The model under review builds one solid part; all positions refer to its coordinate system, in mm. Face numbers are marked on the shaded views. A direction names the side the tool comes from. Coordinates: 2 decimals unless noted, no trailing zeros. Order: outer loops, then holes, each group sorted by start corner. A loop starts at its lowest first (then second) coordinate and runs counter-clockwise, first axis right, second up.
```python
from build123d import *

# Parameters (mm, degrees)
SKETCH_1_R          = 6
EXTRUDE_1_DEPTH     = 20
CUT_EXTRUDE_1_DEPTH = 8
CUT_EXTRUDE_START   = -6
SKETCH_3_R          = 6
SKETCH_3_R_2        = 4.1
CUT_EXTRUDE_2_DEPTH = 6
FILLET_1_R          = 1


with BuildPart() as part:
    # Эскиз1 → Вытянуть1 (new body)
    with BuildSketch(Plane(origin=(0, 0, 0), x_dir=(0, 0, -1), z_dir=(1, 0, 0))):
        Circle(SKETCH_1_R)
    extrude(amount=EXTRUDE_1_DEPTH)

    # Эскиз2 → Вырез-Вытянуть1 (cut)
    with BuildSketch(Plane.ZY):
        Polygon((-3, -1.732050808), (0, -3.464101615), (0, 3.464101615), (-3, 1.732050808), align=None)
        Polygon((0, -3.464101615), (0, 3.464101615), (3, 1.732050808), (3, -1.732050808), align=None)
    extrude(amount=-CUT_EXTRUDE_1_DEPTH, mode=Mode.SUBTRACT)

    # Эскиз3 → Вырез-Вытянуть2 (cut)
    with BuildSketch(Plane(origin=(20, 0, 0), x_dir=(0, 0, -1), z_dir=(1, 0, 0)).offset(CUT_EXTRUDE_START)):
        Circle(SKETCH_3_R)
        Circle(SKETCH_3_R_2, mode=Mode.SUBTRACT)
    extrude(amount=CUT_EXTRUDE_2_DEPTH, mode=Mode.SUBTRACT)

    # Эскиз4 → Вырез-Повернуть1 (revolve, cut)
    with BuildSketch(Plane.XY, mode=Mode.PRIVATE) as cut_revolve_1_sk:
        Polygon((14, 6), (14, 4.1), (12.1, 6), align=None)
    revolve(cut_revolve_1_sk.sketch.rotate(Axis((0, 0, 0), (1, 0, 0)), 90), axis=Axis((0, 0, 0), (1, 0, 0)), mode=Mode.SUBTRACT)

    # Эскиз5 → Вырез-Повернуть2 (revolve, cut)
    with BuildSketch(Plane.XY, mode=Mode.PRIVATE) as cut_revolve_2_sk:
        Polygon((0, 6), (0, 4.9), (1.1, 6), align=None)
    revolve(cut_revolve_2_sk.sketch.rotate(Axis((0, 0, 0), (1, 0, 0)), 90), axis=Axis((0, 0, 0), (1, 0, 0)), mode=Mode.SUBTRACT)

    # Скругление1
    fillet_1_edges = [part.edges().sort_by_distance(p)[0] for p in [
        (8, -2.598076211, 1.5),
        (8, -2.598076211, -1.5),
        (8, 0, -3),
        (8, 2.598076211, -1.5),
        (8, 2.598076211, 1.5),
        (8, 0, 3),
    ]]
    fillet(fillet_1_edges, radius=FILLET_1_R)


solid = part.part
```
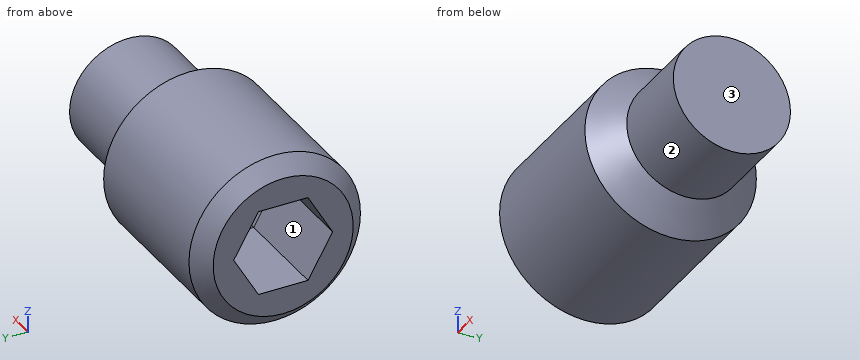
(1) We need section A-A, the plane x = 5.25. Write out the cut boundary in (y, z), and give its area (3 significant figures).
A:
outline: circle Ø12 at (0, 0); hole (-3.46, 0) - (-1.73, -3) - (1.73, -3) - (3.46, 0) - (1.73, 3) - (-1.73, 3) - close
area: 81.9 mm2
(2) We need section C-C, the plane x = 18.25. Write out the cut boundary in (y, z), and give its area (3 significant figures).
A:
outline: circle Ø8.2 at (0, 0)
area: 52.8 mm2
(3) We need section B-B, the plane y = 0. Write out the cut boundary in (x, z).
A:
outline: (0, -4.9) - (1.1, -6) - (12.1, -6) - (14, -4.1) - (20, -4.1) - (20, 4.1) - (14, 4.1) - (12.1, 6) - (1.1, 6) - (0, 4.9) - (0, 3) - (7, 3) arc R1 cw to (8, 2) - (8, -2) arc R1 cw to (7, -3) - (0, -3) - close
(4) Machinability: for the marked faces 1, 2 and 3, which of the approach directions +Z, -Z, +X, -X, +Y, -Y give a long, thin tool a straight path to every point of the face, cutting with its end or side? Answer none if there is none.
A:
face 1: -X
face 2: +X
face 3: +Z, -Z, +X, +Y, -Y
(5) For pin 1 Ø1 at (x, z) = (12, 3) entering from -Y; pin 2 Ø1.5 at (x, y) = (7, -3) entering from +Z; pin 3 Ø5 at (x, y) = (5, -4) entering from -Z, all flat-tipped, find the tip position at first contact; note any pin that passes through.
A:
pin 1: stops at y = -5.45
pin 2: stops at z = 5.56
pin 3: stops at z = -5.81
(6) Wall thickness on probe 1 along Y at (x, z) = (6.25, 1.75); probe 2 along Z at (x, y) = (1, 3); probe 3 along Y at (x, z) = (4.5, -2.75): over which ranges is each line inside the solid? List them lowest first.
A:
probe 1: y = -5.74 to -2.45, 2.45 to 5.74
probe 2: z = -5.08 to -0.8, 0.8 to 5.08
probe 3: y = -5.33 to -1.88, 1.88 to 5.33
